For this review, take the finished solid that the model builds, in its own axes (mm). Face numbers are marked on the shaded views. A direction names the side the tool comes from. Give positions to 0.01 mm unless a question says otherwise; leave off trailing zeros. Write each loop counter-clockwise with the first axis right and the second up, starting at its lowest first coordinate (ties: lowest second). Pieces come first, ordered by that corner, then holes.
Q1. Machinability: for the marked faces 1 and 2, which of the approach directions +Z, -Z, +X, -X, +Y, -Y give a long, thin tool a straight path to every point of the face, cutting with its end or side? Answer none if there is none.
Q2. We need section B-B (y = 0). Write out the cut boundary in (x, z).
Q3. We need section C-C (z = 0.6). Write out the cut boundary in (x, y), then the cut area to 3 significant figures.
Q4. We need section A-A (z = 3.3). Write out the cut boundary in (x, y), then the cut area to 3 significant figures.
Q5. Insertion check: P1, Ø1.5, axis at y = 0.5, z = 2.5, coming from the -X side; P2, Ø1.1, axis at x = -29.5, y = 0, coming from the +Z side. Each pin has a flat end and moves straight along its axis. Give the tip position at first contact, or say it passes through.
Q6. For line 1 (Z direction, x = -14, y = 0.25); line 2 (Y direction, x = -39, z = 3.55); line 3 (Y direction, x = -16, z = 1.3), list the stretches that pass through material, from the lowest coordinate up.
```python
from build123d import *

# Parameters (mm, degrees)
BOSS_EXTRUDE1_DEPTH = 45


with BuildPart() as part:
    # Sketch1 → Boss-Extrude1 (new body)
    with BuildSketch(Plane(origin=(0, 0, 0), x_dir=(0, 0, -1), z_dir=(1, 0, 0))):
        with BuildLine():
            Line((0, 1.752794941), (0, 0))
            Line((0, 0), (1.2, 0))
            Line((1.2, 0), (1.2, 2.25))
            ThreePointArc((1.2, 2.25), (0.204042598, 4.182148799), (-1.79143145, 5.044247083))
            ThreePointArc((-1.79143145, 5.044247083), (-3.03361172, 4.709604832), (-3.814999682, 3.687631197))
            add(Edge.make_bspline(
                [(-3.814999682, 3.687631197), (-4.023588676, 3.069262046), (-4.083460081, 2.438222998), (-3.998734694, 1.823925967)],
                knots=[0.27184632, 0.27184632, 0.27184632, 0.27184632, 0.735422056, 0.735422056, 0.735422056, 0.735422056], degree=3))
            ThreePointArc((-3.998734694, 1.823925967), (-2.034305834, 3.823609616), (0, 1.895056993))
            ThreePointArc((0, 1.895056993), (0.000948954, 1.859497107), (0.001265306, 1.823925967))
            ThreePointArc((0.001265306, 1.823925967), (0.000948954, 1.788354828), (0, 1.752794941))
        make_face()
    extrude(amount=-BOSS_EXTRUDE1_DEPTH)

    # Mirror1: part across plane


with BuildPart() as part_1:
    add(part.part)
    add(part.part.mirror(Plane(origin=(-45, 0, 0), x_dir=(0, 0, 1), z_dir=(0, -1, 0))))


solid = part_1.part
```
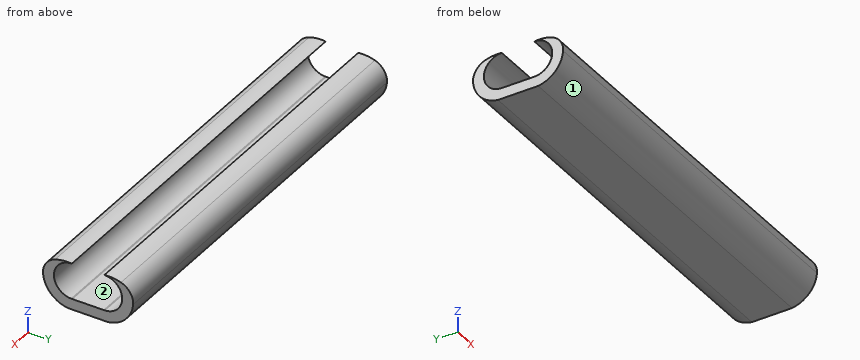
Computed:
1. face 1: -Z, +X, -X, -Y
1. face 2: +Z, +X, -X
2. outline: (-45, -1.2) - (0, -1.2) - (0, 0) - (-45, 0) - close
3. outline: (-45, -4.73) - (0, -4.73) - (0, -3.25) - (-45, -3.25) - close; (-45, 3.25) - (0, 3.25) - (0, 4.73) - (-45, 4.73) - close
3. area: 133 mm2
4. outline: (-45, -4.5) - (0, -4.5) - (0, -3.34) - (-45, -3.34) - close; (-45, 3.34) - (0, 3.34) - (0, 4.5) - (-45, 4.5) - close
4. area: 104 mm2
5. P1: passes through
5. P2: stops at z = 0
6. line 1: z = -1.2 to 0
6. line 2: y = -4.21 to -3.09, 3.09 to 4.21
6. line 3: y = -4.97 to -3.7, 3.7 to 4.97
